from build123d import *

# Parameters (mm, degrees)
SKETCH_1_R          = 1.6
EXTRUDE_1_DEPTH     = 66.6
CUT_EXTRUDE_1_DEPTH = 70.078288919


with BuildPart() as part:
    # 草图1 → 凸台-拉伸1 (new body)
    with BuildSketch(Plane.XY):
        with BuildLine():
            Line((-4, -12.5), (-4, 12.5))
            ThreePointArc((-4, 12.5), (0, 16.5), (4, 12.5))
            Line((4, 12.5), (4, -12.5))
            ThreePointArc((4, -12.5), (0, -16.5), (-4, -12.5))
        make_face()
        with Locations((0, 12.5)):
            Circle(SKETCH_1_R, mode=Mode.SUBTRACT)
        with Locations((0, -12.5)):
            Circle(SKETCH_1_R, mode=Mode.SUBTRACT)
    extrude(amount=EXTRUDE_1_DEPTH)

    # 草图2 → 切除-拉伸1 (cut, through all)
    with BuildSketch(Plane(origin=(4, 0, 0), x_dir=(0, 0, -1), z_dir=(1, 0, 0))):
        with BuildLine():
            Line((-17.8, -6), (-48.8, -6))
            ThreePointArc((-48.8, -6), (-50.214213562, -5.414213562), (-50.8, -4))
            Line((-50.8, -4), (-50.8, 4))
            ThreePointArc((-50.8, 4), (-50.214213562, 5.414213562), (-48.8, 6))
            Line((-48.8, 6), (-17.8, 6))
            ThreePointArc((-17.8, 6), (-16.385786438, 5.414213562), (-15.8, 4))
            Line((-15.8, 4), (-15.8, -4))
            ThreePointArc((-15.8, -4), (-16.385786438, -5.414213562), (-17.8, -6))
        make_face()
    extrude(amount=-CUT_EXTRUDE_1_DEPTH, mode=Mode.SUBTRACT)


solid = part.part
Design review of the part built by this model. Coordinates are the model's own, in mm. A direction names the side the tool comes from. Give positions to 0.01 mm unless a question says otherwise; leave off trailing zeros. Write each loop counter-clockwise with the first axis right and the second up, starting at its lowest first coordinate (ties: lowest second). Pieces come first, ordered by that corner, then holes. Notation, with made-up numbers: M -24,-12.5 L -16,-12.5 A29 ccw -16,17.5 Z; hole C -29.75,27.25 d9. An arc over 180 degrees is marked long. Answer as a JSON object with one key per item and string values. Group by question number.
1) We need section D-D (z = 21). Give the boundary of the cut face in (x, y).
2) We need section B-B (z = 50). Give the boundary of the cut face in (x, y), and give its area (3 significant figures).
3) We need section A-A (x = 0). Give the boundary of the cut face in (y, z).
4) For line 1 along Y through (x, z) = (0, 36.5); line 2 along Z through (x, y) = (-3, 1); line 3 along Y through (x, z) = (1, 19), list the stretches that pass through material, from the lowest coordinate up.
5) Mouldability with a two-part tool opening along Z and no side actions: class faces 3 (the face through (0, 0, 66.6)), 4 (the face through (-0.208, 14.086, 32.834)), 5 (the face through (0, 0, 15.8)), 6 (the face through (0, 0, 0)) as released by +Z, released by -Z, zero draft, split by the parting line, or undercut.
6) Tool access review of faces 1 (the face through (0, 6, 34)), 2 (the face through (-0.1, 16.5, 32.8)): name each direction out of +Z, -Z, +X, -X, +Y, -Y from which nothing blocks a thin tool from reaching the whole face with its end or side.
7) Clearance check with a flat-ended pin moving along its axis: pin 1 Ø1 at (x, z) = (-1, 16) entering from -Y. State where the tip first meets the part, or that it passes through.
8) We need section C-C (y = 1.5). Give the boundary of the cut face in (x, z), and give its area (3 significant figures).
Answer key:
{
 "1": {"outline": "M -4,-12.5 A4 ccw 4,-12.5 L 4,-6 L -4,-6 Z; M -4,6 L 4,6 L 4,12.5 A4 ccw -4,12.5 Z; hole C 0,-12.5 d3.2; hole C 0,12.5 d3.2"},
 "2": {"outline": "M -4,-12.5 A4 ccw 4,-12.5 L 4,-5.6 L -4,-5.6 Z; M -4,5.6 L 4,5.6 L 4,12.5 A4 ccw -4,12.5 Z; hole C 0,-12.5 d3.2; hole C 0,12.5 d3.2", "area": "145 mm²"},
 "3": {"outline": "M -16.5,0 L -14.1,0 L -14.1,66.6 L -16.5,66.6 Z; M -10.9,0 L 10.9,0 L 10.9,66.6 L -10.9,66.6 Z; M 14.1,0 L 16.5,0 L 16.5,66.6 L 14.1,66.6 Z; hole M -6,17.8 A2 ccw -4,15.8 L 4,15.8 A2 ccw 6,17.8 L 6,48.8 A2 ccw 4,50.8 L -4,50.8 A2 ccw -6,48.8 Z"},
 "4": {"line 1": "y = -16.5 to -14.1, -10.9 to -6, 6 to 10.9, 14.1 to 16.5", "line 2": "z = 0 to 15.8, 50.8 to 66.6", "line 3": "y = -16.37 to -13.75, -11.25 to -6, 6 to 11.25, 13.75 to 16.37"},
 "5": {"face 3": "released by +Z", "face 4": "zero draft", "face 5": "undercut", "face 6": "released by -Z"},
 "6": {"face 1": "+X, -X", "face 2": "+Z, -Z, +Y"},
 "7": {"pin 1": "stops at y = -16.47"},
 "8": {"outline": "M -4,0 L 4,0 L 4,15.8 L -4,15.8 Z; M -4,50.8 L 4,50.8 L 4,66.6 L -4,66.6 Z", "area": "253 mm²"}
}
